Autodesk Inventor part; units mm, degrees
ref_plane "YZ Plane" through (0, 0, 0) normal (1, 0, 0) x (0, 1, 0)
ref_plane "XZ Plane" through (0, 0, 0) normal (0, 1, 0) x (-1, 0, 0)
ref_plane "XY Plane" through (0, 0, 0) normal (0, 0, 1) x (1, 0, 0)
sketch "Sketch1" plane through (0, 0, 0) normal (0, 0, 1) x (1, 0, 0)
  line L0 (-14.3448, 13.9006) -> (-7.8021, 17.4592)
  line L1 (-14.3448, 13.9006) -> (-14.5342, 6.4551)
  line L2 (-14.5342, 6.4551) -> (-8.1811, 2.5683)
  line L3 (-8.1811, 2.5683) -> (-1.6384, 6.127)
  line L4 (-1.4489, 13.5724) -> (-1.6384, 6.127)
  line L5 (-7.8021, 17.4592) -> (-1.4489, 13.5724)
  circle A0 centre (-8, 10) radius 4
  circle A1 centre (-8, 10) radius 7.5414
  line L6 (-4.1827, 16.5039) -> (-0.4588, 9.9461)
  line L7 (-0.4588, 9.9461) -> (-4.2761, 3.4422)
  line L8 (-4.2761, 3.4422) -> (-11.8173, 3.4961)
  line L9 (-11.8173, 3.4961) -> (-15.5412, 10.0539)
  line L10 (-15.5412, 10.0539) -> (-11.7239, 16.5578)
  line L11 (-11.7239, 16.5578) -> (-4.1827, 16.5039)
  circle A2 centre (-8, 10) radius 4.25
  circle A3 centre (-8, 10) radius 12.5
  point P0 (0, 0)
extrude "Extrusion1" add sketch "Sketch1" along normal blind 12 contours L1 L10 A1 L0 | L0 L10 L1 | L11 A1 L5 L0 | L0 L5 L11 | L9 L2 L1 | L1 L2 L9 A1 | A1 L6 L4 L5 | L8 L2 L3 A1 | L5 L4 L6 | L8 L3 L2 | L7 L3 L4 A1 | L7 L4 L3 | A3
sketch "Sketch2" plane through (-8, 10, 12) normal (0, 0, 1) x (1, 0, 0)
  circle A0 centre (0, 0) radius 4.25
  line L0 (7.5412, -0.0539) -> (3.7239, -6.5578)
  circle A1 centre (0, 0) radius 7.5414
  point P0 (8, -10)
  dimension "d4" = 8.5
extrude "Extrusion2" add sketch "Sketch2" along normal blind 3
properties part number "gear1"
Source: CAD feature listing. Evaluate the final solid. Frame: model axes, mm. A direction names the side the tool comes from. Coordinates: 2 decimals unless noted, no trailing zeros. Write each loop counter-clockwise with the first axis right and the second up, starting at its lowest first coordinate (ties: lowest second). Pieces come first, ordered by that corner, then holes. Notation, with made-up numbers: M 52,56 L 67,56 A28 ccw 67,75 Z; hole C 57.5,64 d11. An arc over 180 degrees is marked long. Answer as a JSON object with one key per item and string values.
1. Ray query, L1, parallel to Y at x = -8, z = 12.8; L2, parallel to X at y = 6.25, z = 13.5; L3, parallel to Z at x = -6.5, y = -1.5. Return the intervals inside material, ascending.
Evaluation:
{"L1": "2.46 to 5.75, 14.25 to 17.54", "L2": "-14.54 to -10, -6 to -1.46", "L3": "0 to 12"}
2. Access query for faces 1 (the flat face through (-2.34, 6.74, 5.92)), 2 (the cylindrical face through (-11.37, 12.59, 13.48)), 3 (the flat face through (0, 10, 12)). Directions: +Z, -Z, +X, -X, +Y, -Y. A direction counts if a zero-diameter tool reaches every point of the face in a straight line with its end or side. Return the directions, or none.
Evaluation:
{"face 1": "-Z", "face 2": "+Z, -Z", "face 3": "+Z"}
3. Cut plane B-B on x = -5.25. Output: boundary loops of the cut face in (y, z).
Evaluation:
{"outline": "M -2.19,0 L 3.45,0 L 3.45,12 L 6.76,12 L 6.76,15 L 2.98,15 L 2.98,12 L -2.19,12 Z; M 13.24,12 L 16.51,12 L 16.51,0 L 22.19,0 L 22.19,12 L 17.02,12 L 17.02,15 L 13.24,15 Z"}
4. Cut plane D-D on z = 13.75. Output: boundary loops of the cut face in (x, y), plus the area to 3 significant figures.
Evaluation:
{"outline": "C -8,10 d15.08; hole C -8,10 d8.5", "area": "122 mm^2"}
5. Cut plane A-A on z = 10.25. Output: boundary loops of the cut face in (x, y), plus the area to 3 significant figures.
Evaluation:
{"outline": "C -8,10 d25; hole M -15.54,10.05 L -11.82,3.5 L -4.28,3.44 L -0.46,9.95 L -4.18,16.5 L -11.72,16.56 Z", "area": "343 mm^2"}
6. Cut plane C-C on y = 20. Output: boundary loops of the cut face in (x, z).
Evaluation:
{"outline": "M -15.5,0 L -0.5,0 L -0.5,12 L -15.5,12 Z"}
7. Contact query for flat-ended pins moving along their axis: P1, Ø4, axis at y = 2, z = 10, coming from the -X side; P2, Ø8, axis at x = -13.5, z = 10, coming from the +Y side; P3, Ø4, axis at x = -14, z = 1.5, coming from the -Y side. Output: stop coordinate, or through.
Evaluation:
{"P1": "x = -18.97", "P2": "y = 22.41", "P3": "y = -1.84"}
